Source: three-view drawing plus pictorial views. Frame: mm from the lowest corner of the part. A direction names the side the tool comes from. Round coordinates to 2 decimals unless told otherwise and drop trailing zeros. Loops run counter-clockwise (first coordinate to the right, second up) from the corner with the lowest first, then second, coordinate; pieces in that order, holes last. Notation, with made-up numbers: M 7.5,3.25 L 43.5,3.25 A17 cw 43.5,32.25 Z; hole C 53.5,-5.5 d5. An arc over 180 degrees is marked long. Answer as a JSON object with one key per item and string values.
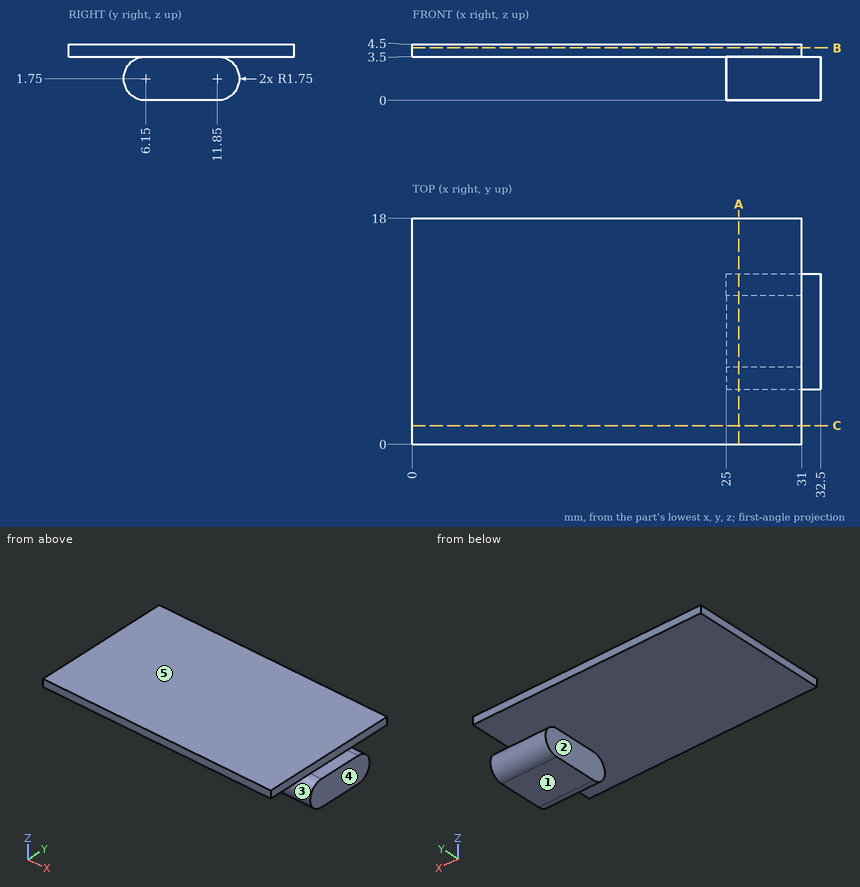
1) Pull-direction query (Z, two-part tool) for the marked faces 3, 4 and 5; classes: +Z half, -Z half, draft (parallel to the pull), parting line (faces both ways), or undercut.
Geometry results:
{"face 3": "undercut", "face 4": "draft", "face 5": "+Z half"}
2) First-contact query: pin 1 (1 mm diameter, centred on y = 12, z = 1.5, fed in from -X); pin 2 (10 mm diameter, centred on x = 10.5, y = 10.5, fed in from -Z). Flat tips, straight axial feed; report the tip coordinate or a pass-through.
Geometry results:
{"pin 1": "x = 25", "pin 2": "z = 3.5"}
3) Line query: probe 1 along X at (y, z) = (5, 3.9); probe 2 along Z at (x, y) = (20, 14.75); probe 3 along X at (y, z) = (6.25, 2.85). Output: solid intervals per line, ascending.
Geometry results:
{"probe 1": "0 to 31", "probe 2": "3.5 to 4.5", "probe 3": "25 to 32.5"}
4) Cut plane C-C on y = 1.5. Return the cut outline in (x, z), and give its area (3 significant figures).
Geometry results:
{"outline": "M 0,3.5 L 31,3.5 L 31,4.5 L 0,4.5 Z", "area": "31.0 mm2"}
5) Set-up query: the marked faces 1 and 2. Return all of +Z, -Z, +X, -X, +Y, -Y with unobstructed straight access to the full face (end or side cutting, diameter ignored); none if empty.
Geometry results:
{"face 1": "-Z, +X, -X, +Y, -Y", "face 2": "-Z, -X, +Y, -Y"}
6) Cut plane B-B on z = 4.2. Return the cut outline in (x, y).
Geometry results:
{"outline": "M 0,0 L 31,0 L 31,18 L 0,18 Z"}
7) Cut plane A-A on x = 26. Return the cut outline in (y, z).
Geometry results:
{"outline": "M 0,3.5 L 6.15,3.5 A1.75 ccw 6.15,0 L 11.85,0 A1.75 ccw 11.85,3.5 L 18,3.5 L 18,4.5 L 0,4.5 Z"}
